from build123d import *

# Parameters (mm, degrees)
SKETCH_1_R          = 23.5
SKETCH_1_R_2        = 17.5
SKETCH_1_R_3        = 16.5
EXTRUDE_1_DEPTH     = 1
SKETCH_2_R          = 23.5
SKETCH_2_R_2        = 17.5
EXTRUDE_2_DEPTH     = 1
SKETCH_3_R          = 1.5
CUT_EXTRUDE_1_DEPTH = 11


with BuildPart() as part:
    # 草图1 → 凸台-拉伸1 (new body)
    # profile 1 of 2: a face of its own
    with BuildSketch(Plane(origin=(0, 0, 0), x_dir=(1, 0, 0), z_dir=(0, 1, 0))):
        with Locations(Location((0, 0, 0), (0, 0, 270))):
            Circle(SKETCH_1_R)
        Circle(SKETCH_1_R_2, mode=Mode.SUBTRACT)
    # profile 2 of 2: a face of its own
    with BuildSketch(Plane(origin=(0, 0, 0), x_dir=(1, 0, 0), z_dir=(0, 1, 0))):
        Circle(SKETCH_1_R_2)
        with Locations(Location((0, 0, 0), (0, 0, 270))):
            Circle(SKETCH_1_R_3, mode=Mode.SUBTRACT)
    extrude(amount=EXTRUDE_1_DEPTH)

    # 草图2 → 凸台-拉伸2 (add)
    with BuildSketch(Plane(origin=(0, 1, 0), x_dir=(1, 0, 0), z_dir=(0, 1, 0))):
        with Locations(Location((0, 0, 0), (0, 0, 270))):
            Circle(SKETCH_2_R)
        with Locations(Location((0, 0, 0), (0, 0, 270))):
            Circle(SKETCH_2_R_2, mode=Mode.SUBTRACT)
    extrude(amount=EXTRUDE_2_DEPTH)

    # 草图3 → 切除-拉伸1 (cut)
    with BuildSketch(Plane(origin=(0, 2, 0), x_dir=(1, 0, 0), z_dir=(0, 1, 0))):
        with Locations(Location((0, 20.5, 0), (0, 0, 270))):
            Circle(SKETCH_3_R)
        with Locations(Location((20.5, 0, 0), (0, 0, 270))):
            Circle(SKETCH_3_R)
        with Locations(Location((0, -20.5, 0), (0, 0, 270))):
            Circle(SKETCH_3_R)
        with Locations(Location((-20.5, 0, 0), (0, 0, 270))):
            Circle(SKETCH_3_R)
    extrude(amount=-CUT_EXTRUDE_1_DEPTH, mode=Mode.SUBTRACT)


solid = part.part
Geometry: final body of the model. Coordinates: model frame, mm. A direction names the side the tool comes from. Round coordinates to 2 decimals unless told otherwise and drop trailing zeros. Order: outer loops, then holes, each group sorted by start corner. A loop starts at its lowest first (then second) coordinate and runs counter-clockwise, first axis right, second up. Notation, with made-up numbers: (68, 88.25) -> (84, 88.25) arc R19 ccw to (84, 125.25) -> close; hole circle Ø4 at (-6, -34.5). An arc over 180 degrees is marked (long way). Put each result on its own line as item: value. Start each with the question number.
Q1. First-contact query: pin 1 (1 mm diameter, centred on x = -15, z = 4, fed in from -Y). Flat tip, straight axial feed; report the tip coordinate or a pass-through.
Q2. Section C-C on y = 0.6. Return the cut outline in (x, z), and give its area (3 significant figures).
Q3. Reachability of faces 1 (the cylindrical face through (-10.648, 1.493, -13.887)), 2 (the cylindrical face through (-19.235, 1.014, 0.806)) from +Z, -Z, +X, -X, +Y, -Y: full face, straight path, thin tool, end or side. Return the list, or none.
Q4. Section B-B on x = 0. Return the cut outline in (y, z), and give its area (3 significant figures).
Q5. Pull-direction query (Z, two-part tool) for faces 3 (the flat face through (-16, 1, -5)), 4 (the cylindrical face through (15.88, 0.99, -17.32)), 5 (the flat face through (-12, 0, 12)); classes: +Z half, -Z half, draft (parallel to the pull), parting line (faces both ways), or undercut.
Q6. Section A-A on z = 0. Return the cut outline in (x, y), and give its area (3 significant figures).
Q7. Section D-D on z = -12.5. Return the cut outline in (x, y), and give its area (3 significant figures).
Q8. Line query: probe 1 along X at (y, z) = (0.7, 0); probe 2 along X at (y, z) = (1.55, 0); probe 3 along X at (y, z) = (0.55, -7). Output: solid intervals per line, ascending.
Ans:
1. pin 1: passes through
2. outline: circle Ø47 at (0, 0); hole circle Ø3 at (-20.5, 0); hole circle Ø33 at (0, 0); hole circle Ø3 at (0, -20.5); hole circle Ø3 at (0, 20.5); hole circle Ø3 at (20.5, 0)
2. area: 851 mm2
3. face 1: +Y
3. face 2: +Y, -Y
4. outline: (0, -23.5) -> (2, -23.5) -> (2, -22) -> (0, -22) -> close; (0, -19) -> (2, -19) -> (2, -17.5) -> (1, -17.5) -> (1, -16.5) -> (0, -16.5) -> close; (0, 16.5) -> (1, 16.5) -> (1, 17.5) -> (2, 17.5) -> (2, 19) -> (0, 19) -> close; (0, 22) -> (2, 22) -> (2, 23.5) -> (0, 23.5) -> close
4. area: 14.0 mm2
5. face 3: undercut
5. face 4: parting line
5. face 5: draft
6. outline: (-23.5, 0) -> (-22, 0) -> (-22, 2) -> (-23.5, 2) -> close; (-19, 0) -> (-16.5, 0) -> (-16.5, 1) -> (-17.5, 1) -> (-17.5, 2) -> (-19, 2) -> close; (16.5, 0) -> (19, 0) -> (19, 2) -> (17.5, 2) -> (17.5, 1) -> (16.5, 1) -> close; (22, 0) -> (23.5, 0) -> (23.5, 2) -> (22, 2) -> close
6. area: 14.0 mm2
7. outline: (-19.9, 0) -> (-10.77, 0) -> (-10.77, 1) -> (-12.25, 1) -> (-12.25, 2) -> (-19.9, 2) -> close; (10.77, 0) -> (19.9, 0) -> (19.9, 2) -> (12.25, 2) -> (12.25, 1) -> (10.77, 1) -> close
7. area: 33.6 mm2
8. probe 1: x = -23.5 to -22, -19 to -16.5, 16.5 to 19, 22 to 23.5
8. probe 2: x = -23.5 to -22, -19 to -17.5, 17.5 to 19, 22 to 23.5
8. probe 3: x = -22.43 to -14.94, 14.94 to 22.43
